Here's the drawing with two shaded views (mm, measured from the low corner). I have some questions. Give positions to 0.01 mm unless a question says otherwise; leave off trailing zeros. Order: outer loops, then holes, each group sorted by start corner. A loop starts at its lowest first (then second) coordinate and runs counter-clockwise, first axis right, second up. Notation, with made-up numbers: M 16,22.25 L 57,22.25 A25 ccw 57,39.25 Z; hole C 21.5,56.25 d8. An arc over 180 degrees is marked long. Write each question's results on one line, items separated by ' | '.
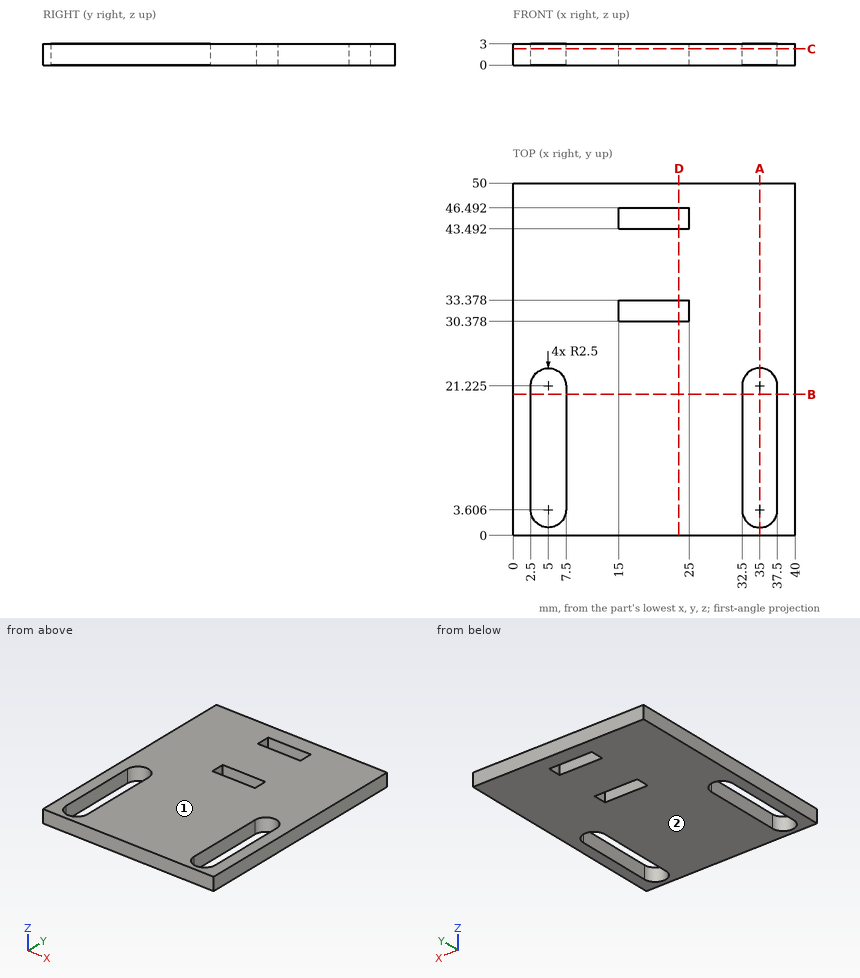
(1) Imagine slicing it at C-C, the plane z = 2.3. Write out the boundary of the cut face in (x, y) (1 decimal).
Data:
outline: M 0,0 L 40,0 L 40,50 L 0,50 Z; hole M 2.5,3.6 A2.5 ccw 7.5,3.6 L 7.5,21.2 A2.5 ccw 2.5,21.2 Z; hole M 15,30.4 L 25,30.4 L 25,33.4 L 15,33.4 Z; hole M 15,43.5 L 25,43.5 L 25,46.5 L 15,46.5 Z; hole M 32.5,3.6 A2.5 ccw 37.5,3.6 L 37.5,21.2 A2.5 ccw 32.5,21.2 Z
(2) Imagine slicing it at D-D, the plane x = 23.5. Write out the boundary of the cut face in (y, z), plus the area to 3 significant figures.
Data:
outline: M 0,0 L 30.38,0 L 30.38,3 L 0,3 Z; M 33.38,0 L 43.49,0 L 43.49,3 L 33.38,3 Z; M 46.49,0 L 50,0 L 50,3 L 46.49,3 Z | area: 132 mm2
(3) Imagine slicing it at B-B, the plane y = 20. Write out the boundary of the cut face in (x, z), plus the area to 3 significant figures.
Data:
outline: M 0,0 L 2.5,0 L 2.5,3 L 0,3 Z; M 7.5,0 L 32.5,0 L 32.5,3 L 7.5,3 Z; M 37.5,0 L 40,0 L 40,3 L 37.5,3 Z | area: 90.0 mm2
(4) I need wall thicknesses on L1, parallel to Y at x = 24, z = 1; L2, parallel to X at y = 9.5, z = 2.05; L3, parallel to X at y = 3, z = 0.7 (1 decimal). Which ranges of each line are inside material? Lowest first, please. Write a range as from..to.
Data:
L1: y = 0..30.38, 33.38..43.49, 46.49..50 | L2: x = 0..2.5, 7.5..32.5, 37.5..40 | L3: x = 0..2.6, 7.4..32.6, 37.4..40
(5) Imagine slicing it at A-A, the plane x = 35. Write out the boundary of the cut face in (y, z) (1 decimal).
Data:
outline: M 0,0 L 1.1,0 L 1.1,3 L 0,3 Z; M 23.7,0 L 50,0 L 50,3 L 23.7,3 Z
(6) We'd pull the mould along Z, two halves only. Please class the marked faces 1 and 2: +Z half, -Z half, draft (parallel to the pull), parting line (faces both ways), or undercut.
Data:
face 1: +Z half | face 2: -Z half
